Design review of the part built by this model. Coordinates are the model's own, in mm. A direction names the side the tool comes from. Give positions to 0.01 mm unless a question says otherwise; leave off trailing zeros. Loops run counter-clockwise (first coordinate to the right, second up) from the corner with the lowest first, then second, coordinate; pieces in that order, holes last. Notation, with made-up numbers: M -26,-1 L -2,-1 A3 ccw -2,4 Z; hole C 83,75.25 d3. An arc over 180 degrees is marked long. Answer as CSV lines item,"result".
```python
from build123d import *

# Parameters (mm, degrees)
BOSS_EXTRUDE1_DEPTH = 3.3
CHAMFER1_SIZE       = 2
SKETCH2_R           = 1.625
CUT_EXTRUDE1_DEPTH  = 2


with BuildPart() as part:
    # Sketch1 → Boss-Extrude1 (new body)
    with BuildSketch(Plane(origin=(0, 0, 0), x_dir=(1, 0, 0), z_dir=(0, 1, 0))):
        with BuildLine():
            Line((-17.971705397, 32.627906846), (-13.729256498, 25.279769804))
            ThreePointArc((-13.729256498, 25.279769804), (0, 28.767329478), (13.729256498, 25.279769804))
            Line((13.729256498, 25.279769804), (17.971705397, 32.627906846))
            ThreePointArc((17.971705397, 32.627906846), (0, 37.25), (-17.971705397, 32.627906846))
        make_face()
    extrude(amount=BOSS_EXTRUDE1_DEPTH)

    # Chamfer1
    chamfer1_edges = [part.edges().sort_by_distance(p)[0] for p in [
        (0, 3.3, -28.767329478),
        (15.850480947, 3.3, -28.953838325),
        (0, 3.3, -37.25),
        (-15.850480947, 3.3, -28.953838325),
    ]]
    chamfer(chamfer1_edges, length=CHAMFER1_SIZE)

    # Sketch2 → Cut-Extrude1 (cut)
    with BuildSketch(Plane.XZ):
        with Locations(Location((0, -33.008664739, 0), (0, 0, 270))):
            Circle(SKETCH2_R)
    extrude(amount=-CUT_EXTRUDE1_DEPTH, mode=Mode.SUBTRACT)


solid = part.part
```
1. We need section A-A, the plane x = 0. Write out the cut boundary in (y, z).
Answer block:
outline,"M 0,-37.25 L 1.3,-37.25 L 3.3,-35.25 L 3.3,-30.77 L 1.3,-28.77 L 0,-28.77 L 0,-31.38 L 2,-31.38 L 2,-34.63 L 0,-34.63 Z"
2. The part is to be moulded in two halves that separate along X. For faces 1 (the flat face through (15.82, 0.64, -28.9)), 2 (the conical face through (-0.203, 1.647, -29.114)), 3 (the flat face through (0, 0, -31)), 4 (the cylindrical face through (0.26, 0.64, -37.25)), say which applies: pulls with the +X half, pulls with the -X half, needs draft (parallel to the pull), parting line crosses it, or undercut.
Answer block:
face 1,"pulls with the +X half"
face 2,"undercut"
face 3,"needs draft"
face 4,"parting line crosses it"
3. For P1, Ø1, axis at x = 13, y = 2, coming from the +Z side; P2, Ø2.5, axis at x = 0, z = -33, coming from the -Y side; P3, Ø1.5, axis at y = 0.5, z = -31.5, coming from the -X side, all flat-tipped, find the tip position at first contact; note any pin that passes through.
Answer block:
P1,"z = -25.83"
P2,"y = 2"
P3,"x = -17.75"
4. To check wall thickness, follow L1, parallel to Y at x = -0.5, z = -31.5; L2, parallel to X at y = 0.65, z = -32.75; L3, parallel to Z at x = 1, y = 1.2. State the ranges of each line that lie inside material, in increasing order. Write a range as [from, to].
Answer block:
L1,"[2, 3.3]"
L2,"[-17.75, -1.6], [1.6, 17.75]"
L3,"[-37.24, -34.29], [-31.73, -28.75]"
5. For faces 5 (the flat face through (0, 2, -33)), 6 (the flat face through (0, 3.3, -32)), list the 3-axis set-ups (+Z, -Z, +X, -X, +Y, -Y) from which the entire face can be reached by the end or side of a thin tool; tool diameter is ignored.
Answer block:
face 5,"-Y"
face 6,"+Z, -Z, +X, -X, +Y"
6. We need section B-B, the plane y = 2.75. Write out the cut boundary in (x, z), plus the area to 3 significant figures.
Answer block:
outline,"M -15.96,-32.05 A35.8 ccw 15.96,-32.05 L 13.16,-27.2 A30.22 cw -13.16,-27.2 Z"
area,"168 mm²"
